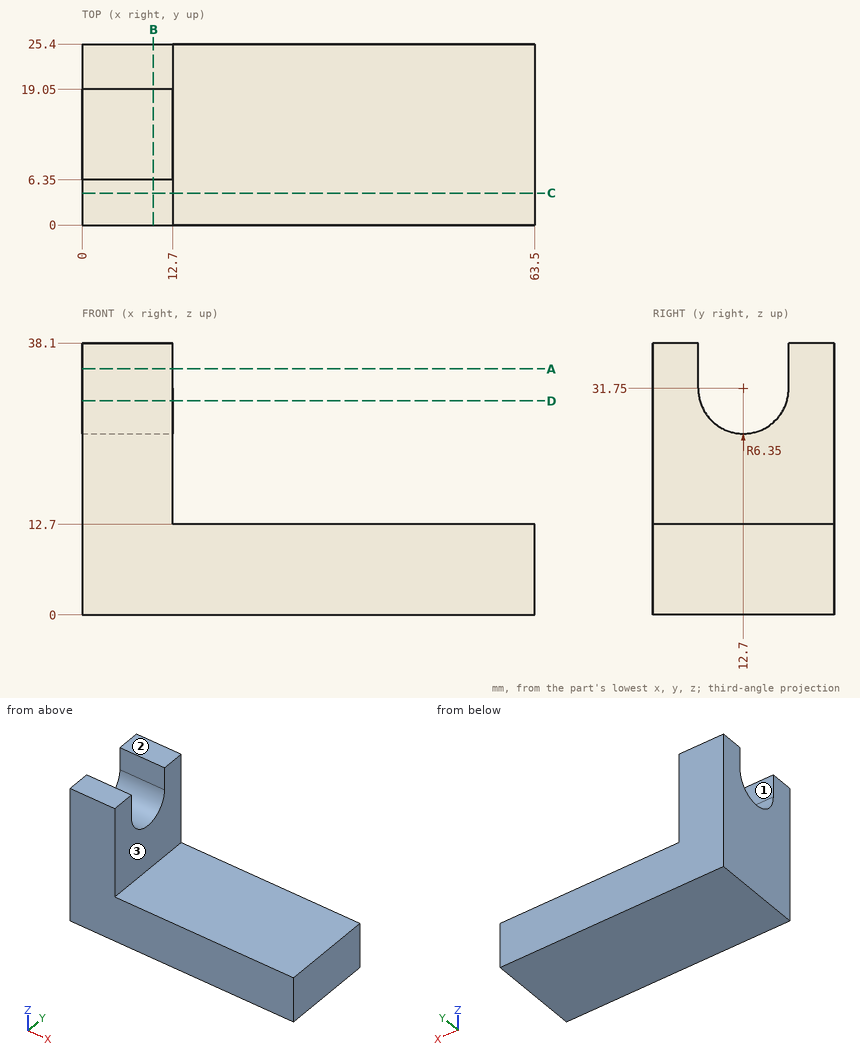
Study the drawing (mm; zero at the part's minimum x, y, z) and answer. A direction names the side the tool comes from. Coordinates: 2 decimals unless noted, no trailing zeros. Write each loop counter-clockwise with the first axis right and the second up, starting at its lowest first coordinate (ties: lowest second). Pieces come first, ordered by that corner, then holes. Notation, with made-up numbers: M -25.5,56 L -12.5,56 A26 ccw -12.5,74 Z; hole C -21.75,50 d1. An arc over 180 degrees is marked long. Write each question's results on one line, items separated by ' | '.
Item 1: The part is cut by section C-C on y = 4.5. Determine the outline of the cut face in (x, z), and give its area (3 significant figures).
Answer below:
outline: M 0,0 L 63.5,0 L 63.5,12.7 L 12.7,12.7 L 12.7,38.1 L 0,38.1 Z | area: 1,130 mm2
Item 2: Which of the six approach directions +Z, -Z, +X, -X, +Y, -Y give full straight-line access (tool end or side, diameter ignored) to the marked faces 1, 2 and 3?
Answer below:
face 1: +Z, +X, -X | face 2: +Z, +X, -X, +Y, -Y | face 3: +Z, +X, +Y, -Y
Item 3: Given P1, Ø2, axis at x = 41.5, y = 21.5, coming from the +Z side; P2, Ø7.5, axis at y = 7, z = 20.5, coming from the +X side; P3, Ø2, axis at y = 19, z = 23, coming from the -X side, each flat-ended and moving along its own axis, determine where each tip first touches the part or whether it passes through.
Answer below:
P1: z = 12.7 | P2: x = 12.7 | P3: x = 0
Item 4: Consider probe 1 along Z at (x, y) = (53.5, 6.5); probe 2 along Z at (x, y) = (7, 18). Determine where each line is inside the solid, lowest interval first. Write a range as [from, to].
Answer below:
probe 1: [0, 12.7] | probe 2: [0, 28.25]
Item 5: The part is cut by section B-B on x = 10. Determine the outline of the cut face in (y, z), and give its area (3 significant figures).
Answer below:
outline: M 0,0 L 25.4,0 L 25.4,38.1 L 19.05,38.1 L 19.05,31.75 A6.35 cw 6.35,31.75 L 6.35,38.1 L 0,38.1 Z | area: 824 mm2
Item 6: The part is cut by section A-A on z = 34.5. Determine the outline of the cut face in (x, y), and give its area (3 significant figures).
Answer below:
outline: M 0,0 L 12.7,0 L 12.7,6.35 L 0,6.35 Z; M 0,19.05 L 12.7,19.05 L 12.7,25.4 L 0,25.4 Z | area: 161 mm2
Item 7: The part is cut by section D-D on z = 30. Determine the outline of the cut face in (x, y).
Answer below:
outline: M 0,0 L 12.7,0 L 12.7,6.6 L 0,6.6 Z; M 0,18.8 L 12.7,18.8 L 12.7,25.4 L 0,25.4 Z
